The drawing under review shows one solid part. Ordinate dimensions are in mm from its lowest x, y, z. A direction names the side the tool comes from. Give positions to 0.01 mm unless a question says otherwise; leave off trailing zeros. Loops run counter-clockwise (first coordinate to the right, second up) from the corner with the lowest first, then second, coordinate; pieces in that order, holes last. Notation, with made-up numbers: (21.25, 32.5) -> (50.25, 32.5) arc R22 ccw to (50.25, 49.5) -> close; hole circle Ø8 at (21, 10). An arc over 180 degrees is marked (long way). Answer in a Markdown table with one row per item. Add a question column.
(1) Consider section B-B on z = 14. Write out the cut boundary in (x, y).
(2) Consider section A-A on y = 58.27. Write out the cut boundary in (x, z).
(3) For line 1 (X direction, y = 23, z = 5); line 2 (Y direction, x = 98.95, z = 14); line 3 (Z direction, x = 96, y = 38), list the stretches that pass through material, from the lowest coordinate up.
(4) For the marked faces 1 and 2, list the 3-axis set-ups (+Z, -Z, +X, -X, +Y, -Y) from which the entire face can be reached by the end or side of a thin tool; tool diameter is ignored.
(5) Consider section D-D on y = 49. Write out the cut boundary in (x, z).
(6) Consider section C-C on x = 96. Write out the cut boundary in (y, z).
(7) For pin 1 (2.5 mm diameter, centred on y = 13.27, z = 14, fed in from +X); pin 2 (1 mm diameter, centred on x = 29, y = 11, fed in from +Z); pin 3 (5 mm diameter, centred on x = 28, y = 3, fed in from +Z), all flat-tipped, find the tip position at first contact; note any pin that passes through.
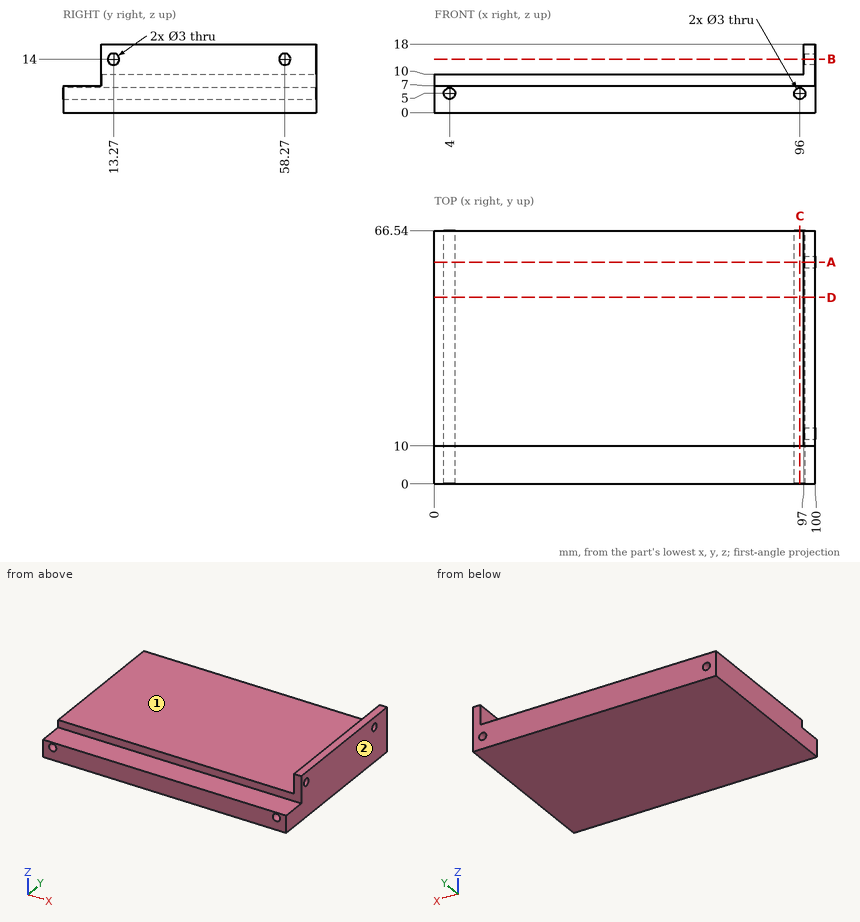
Values follow:
| question | item | result |
|---|---|---|
| 1 | outline | (97, 10) -> (100, 10) -> (100, 11.77) -> (97, 11.77) -> close; (97, 14.77) -> (100, 14.77) -> (100, 56.77) -> (97, 56.77) -> close; (97, 59.77) -> (100, 59.77) -> (100, 66.54) -> (97, 66.54) -> close |
| 2 | outline | (0, 0) -> (100, 0) -> (100, 12.5) -> (97, 12.5) -> (97, 10) -> (0, 10) -> close; (97, 15.5) -> (100, 15.5) -> (100, 18) -> (97, 18) -> close; hole circle Ø3 at (4, 5); hole circle Ø3 at (96, 5) |
| 3 | line 1 | 0 to 2.5, 5.5 to 94.5, 97.5 to 100 |
| 3 | line 2 | 10 to 11.77, 14.77 to 56.77, 59.77 to 66.54 |
| 3 | line 3 | 0 to 3.5, 6.5 to 10 |
| 4 | face 1 | +Z, -X, +Y, -Y |
| 4 | face 2 | +Z, -Z, +X, +Y, -Y |
| 5 | outline | (0, 0) -> (100, 0) -> (100, 18) -> (97, 18) -> (97, 10) -> (0, 10) -> close; hole circle Ø3 at (4, 5); hole circle Ø3 at (96, 5) |
| 6 | outline | (0, 0) -> (66.54, 0) -> (66.54, 3.5) -> (0, 3.5) -> close; (0, 6.5) -> (66.54, 6.5) -> (66.54, 10) -> (10, 10) -> (10, 7) -> (0, 7) -> close |
| 7 | pin 1 | through |
| 7 | pin 2 | z = 10 |
| 7 | pin 3 | z = 7 |
